```python
from build123d import *

# Parameters (mm, degrees)
SKETCH_1_W          = 57
SKETCH_1_H          = 57
EXTRUDE_1_DEPTH     = 76
SKETCH_2_R          = 12
CUT_EXTRUDE_1_DEPTH = 49
SKETCH_3_R          = 2.5
CUT_EXTRUDE_2_DEPTH = 87.026158812
SKETCH_4_R          = 19
EXTRUDE_2_DEPTH     = 1.6
SKETCH_5_R          = 4
EXTRUDE_3_DEPTH     = 18.4
SKETCH_6_W          = 13.034699884
SKETCH_6_H          = 1
CUT_EXTRUDE_3_DEPTH = 15


with BuildPart() as part:
    # 草图1 → 凸台-拉伸1 (new body)
    with BuildSketch(Plane.XY):
        Rectangle(SKETCH_1_W, SKETCH_1_H)
    extrude(amount=EXTRUDE_1_DEPTH)

    # 草图2 → 切除-拉伸1 (cut)
    with BuildSketch(Plane.XY.offset(76)):
        with Locations((-28.5, 28.5)):
            Circle(SKETCH_2_R)
        with Locations((28.5, 28.5)):
            Circle(SKETCH_2_R)
        with Locations((-28.5, -28.5)):
            Circle(SKETCH_2_R)
        with Locations((28.5, -28.5)):
            Circle(SKETCH_2_R)
    extrude(amount=-CUT_EXTRUDE_1_DEPTH, mode=Mode.SUBTRACT)

    # 草图3 → 切除-拉伸2 (cut, through all)
    with BuildSketch(Plane(origin=(0, 0, 0), x_dir=(-1, 0, 0), z_dir=(0, 0, -1))):
        with Locations((-23.5, 23.5)):
            Circle(SKETCH_3_R)
        with Locations((23.5, 23.5)):
            Circle(SKETCH_3_R)
        with Locations((-23.5, -23.5)):
            Circle(SKETCH_3_R)
        with Locations((23.5, -23.5)):
            Circle(SKETCH_3_R)
    extrude(amount=-CUT_EXTRUDE_2_DEPTH, mode=Mode.SUBTRACT)

    # 草图4 → 凸台-拉伸2 (add)
    with BuildSketch(Plane(origin=(0, 0, 0), x_dir=(-1, 0, 0), z_dir=(0, 0, -1))):
        Circle(SKETCH_4_R)
    extrude(amount=EXTRUDE_2_DEPTH)

    # 草图5 → 凸台-拉伸3 (add)
    with BuildSketch(Plane(origin=(0, 0, -1.6), x_dir=(-1, 0, 0), z_dir=(0, 0, -1))):
        Circle(SKETCH_5_R)
    extrude(amount=EXTRUDE_3_DEPTH)

    # 草图6 → 切除-拉伸3 (cut)
    with BuildSketch(Plane(origin=(0, 0, -20), x_dir=(-1, 0, 0), z_dir=(0, 0, -1))):
        with Locations((0, 4)):
            Rectangle(SKETCH_6_W, SKETCH_6_H)
    extrude(amount=-CUT_EXTRUDE_3_DEPTH, mode=Mode.SUBTRACT)


solid = part.part
```
Can you work these out from the model? Positions are in its coordinate system, mm. A direction names the side the tool comes from. Coordinates: 2 decimals unless noted, no trailing zeros. Loops run counter-clockwise (first coordinate to the right, second up) from the corner with the lowest first, then second, coordinate; pieces in that order, holes last. Notation, with made-up numbers: M 5.5,7.25 L 16.5,7.25 A35 ccw 16.5,39.25 Z; hole C 69,-27.75 d2. An arc over 180 degrees is marked long. Put each result on its own line as item: value. Start each with the question number.
(1) Which directions (+Z, -Z, +X, -X, +Y, -Y) give clear straight access to the entire face, cutting with the end or side of a thin tool? Please do faces 4 (the face through (-19.92, -20.11, 51.84)), 5 (the face through (0.867, -3.905, -10.671)), 6 (the face through (19.92, 20.11, 51.84)).
(2) Will these pins go through, and if not, where does the flat tip stop? pin 1 Ø3 at (x, y) = (-23.5, -23.5) entering from -Z; pin 2 Ø6.5 at (x, y) = (23.5, 23.5) entering from +Z; pin 3 Ø2 at (x, z) = (-19.5, 56.5) entering from -Y; pin 4 Ø4.5 at (x, z) = (0.5, -12) entering from +Y.
(3) I need wall thicknesses on probe 1 along Y at (x, z) = (23.5, 10.5); probe 2 along Y at (x, z) = (-23, 9). Which ranges of each line are inside material? Lowest first, please.
(4) Imagine slicing it at D-D on z = 63.5. List the corners of the cut face in (x, y) for me, and give its area (3 significant figures).
(5) Imagine slicing it at B-B on x = 23.5. List the corners of the cut face in (y, z) for me.
(6) Imagine slicing it at C-C on y = 0. List the corners of the cut face in (x, z) for me.
(7) We'd pull the mould along X, two halves only. Please class faces 1 (the face through (0, 0, -20)), 2 (the face through (25.34, 25.19, 13.31)), 3 (the face through (-20.11, 19.92, 51.84)): +X half, -X half, draft (parallel to the pull), parting line (faces both ways), or undercut.
(8) Imagine slicing it at A-A on z = 21.5. List the corners of the cut face in (x, y) for me, and give its area (3 significant figures).
Worked answers:
1. face 4: +Z, -X, -Y
1. face 5: -Z
1. face 6: +Z, +X, +Y
2. pin 1: passes through
2. pin 2: stops at z = 27
2. pin 3: stops at y = -21.87
2. pin 4: stops at y = 3.5
3. probe 1: y = -28.5 to -26, -21 to 21, 26 to 28.5
3. probe 2: y = -28.5 to -25.95, -21.05 to 21.05, 25.95 to 28.5
4. outline: M -28.5,-16.5 A12 cw -16.5,-28.5 L 16.5,-28.5 A12 cw 28.5,-16.5 L 28.5,16.5 A12 cw 16.5,28.5 L -16.5,28.5 A12 cw -28.5,16.5 Z
4. area: 2,800 mm2
5. outline: M -28.5,0 L -26,0 L -26,27 L -28.5,27 Z; M -21,0 L 21,0 L 21,27 L 17.59,27 L 17.59,76 L -17.59,76 L -17.59,27 L -21,27 Z; M 26,0 L 28.5,0 L 28.5,27 L 26,27 Z
6. outline: M -28.5,0 L -19,0 L -19,-1.6 L -4,-1.6 L -4,-20 L 4,-20 L 4,-1.6 L 19,-1.6 L 19,0 L 28.5,0 L 28.5,76 L -28.5,76 Z
7. face 1: draft
7. face 2: undercut
7. face 3: -X half
8. outline: M -28.5,-28.5 L 28.5,-28.5 L 28.5,28.5 L -28.5,28.5 Z; hole C -23.5,-23.5 d5; hole C -23.5,23.5 d5; hole C 23.5,-23.5 d5; hole C 23.5,23.5 d5
8. area: 3,170 mm2
